CAD build for the part. Positions are in the model's coordinates, mm. Round coordinates to 2 decimals unless told otherwise and drop trailing zeros. Loops run counter-clockwise (first coordinate to the right, second up) from the corner with the lowest first, then second, coordinate; pieces in that order, holes last. Notation, with made-up numbers: M 70.5,-9 L 112.5,-9 A15 cw 112.5,6 Z; hole C 60.25,41 d3. An arc over 180 degrees is marked long. Use one line per item in the form item = value.
from build123d import *

# Parameters (mm, degrees)
F0_W     = 150
F0_H     = 10
F1_DEPTH = 5
F2_R     = 1.5
F3_DEPTH = 8


with BuildPart() as f1:
    # F0 (on Front) → F1 (new body, symmetric)
    with BuildSketch(Plane.XZ):
        Rectangle(F0_W, F0_H)
    extrude(amount=F1_DEPTH, both=True)

    # F2 (on face) → F3 (cut)
    with BuildSketch(Plane(origin=(0, 0, -5), x_dir=(1, 0, 0), z_dir=(0, 0, -1))):
        with Locations((72, 0)):
            Circle(F2_R)
        with Locations((58, 0)):
            Circle(F2_R)
    extrude(amount=-F3_DEPTH, mode=Mode.SUBTRACT)


solid = f1.part
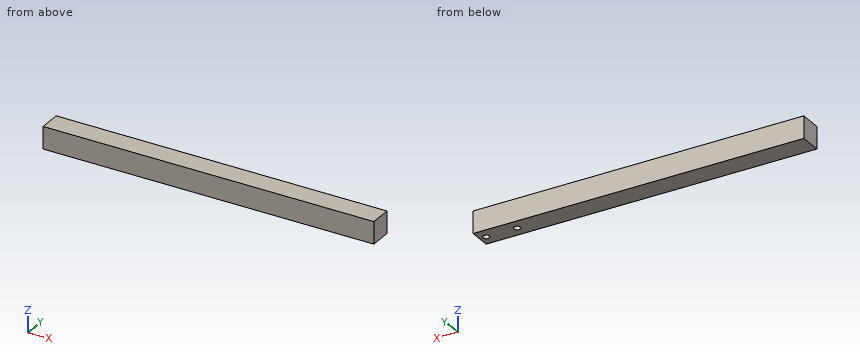
1. Drop a flat-ended pin along its axis: P1, Ø0.9, axis at x = 58, y = 0, coming from the -Z side. Give the stop position or say it passes through.
Completed:
P1 = 3
2. Cut at B-B on y = 0. Write the cut outline in (x, z), and give its area (3 significant figures).
Completed:
outline = M -75,-5 L 56.5,-5 L 56.5,3 L 59.5,3 L 59.5,-5 L 70.5,-5 L 70.5,3 L 73.5,3 L 73.5,-5 L 75,-5 L 75,5 L -75,5 Z
area = 1,450 mm2
3. Cut at A-A on x = 72. Write the cut outline in (y, z).
Completed:
outline = M -5,-5 L -1.5,-5 L -1.5,3 L 1.5,3 L 1.5,-5 L 5,-5 L 5,5 L -5,5 Z
4. Probe line 1 along X through (y, z) = (0, -2); line 2 along X through (y, z) = (1.25, -3.25); line 3 along Y through (x, z) = (58, -1.5). List the from-to ranges inside material, lowest first. Write a range as from..to.
Completed:
line_1 = -75..56.5, 59.5..70.5, 73.5..75
line_2 = -75..57.17, 58.83..71.17, 72.83..75
line_3 = -5..-1.5, 1.5..5
